The listing builds one solid part. Answer for the finished solid, in the listing's coordinates (mm). A direction names the side the tool comes from. Round coordinates to 2 decimals unless told otherwise and drop trailing zeros. Write each loop counter-clockwise with the first axis right and the second up, starting at its lowest first coordinate (ties: lowest second). Pieces come first, ordered by that corner, then holes. Notation, with made-up numbers: (34, 23) - (75, 23) arc R8 cw to (75, 38) - close; hole circle Ø2 at (18.25, 48). An arc over 180 degrees is marked (long way). Return JSON: item names as keys, results as strings. Group by question number.
(1) Each of these flat-tipped pins is pushed along its axis until it touches: pin 1 (2 mm diameter, centred on y = 131, z = 19, fed in from -X); pin 2 (5 mm diameter, centred on x = -15, z = 11.5, fed in from +Y); pin 3 (2 mm diameter, centred on x = -1.5, y = 134, fed in from -Z). Where does it stop, or does it pass through?
(2) Section A-A, the plane y = 120.5 is taken. Write down the section's boundary in (x, z).
(3) Which of the six approach directions +Z, -Z, +X, -X, +Y, -Y give full straight-line access (tool end or side, diameter ignored) to faces 4 (the flat face through (-16.028, 127.352, -1.676)), 5 (the cylindrical face through (-19.76, 136.28, -8.27)), 6 (the flat face through (-6.8, 127.5, 14.2))?
(4) Section B-B, the plane z = -0.5 is taken. Write down the section's boundary in (x, y).
(5) Determine the mould class of faces 1 (the cylindrical face through (-1, 120, 24)), 2 (the cylindrical face through (0.08, 119.36, 26.1)), 3 (the flat face through (-12, 136.799, 6)) for opening direction X: +X half, -X half, draft (parallel to the pull), parting line (faces both ways), or undercut.
(6) Section C-C, the plane y = 126.5 is taken. Write down the section's boundary in (x, z), then the cut area to 3 significant figures.
(7) Find the intervals of material crossed by line 1 along Y through (x, z) = (-17, -2); line 2 along X through (y, z) = (123.25, -8.5); line 3 along Y through (x, z) = (-19.25, -6), in increasing order. Write a range as [from, to].
(8) Section D-D, the plane x = -8.75 is taken. Write down the section's boundary in (y, z).
```python
from build123d import *

# Parameters (mm, degrees)
SKETCH1_R           = 2.15
BOSS_EXTRUDE1_DEPTH = 4.45
FILLET1_R           = 3


with BuildPart() as part:
    # Sketch1 → Boss-Extrude1 (new body)
    with BuildSketch(Plane(origin=(-13.195504222, 0, 7.618427915), x_dir=(0.5, 0, 0.866025404), z_dir=(-0.866025404, 0, 0.5))):
        Polygon((-25.134165871, 118.055853922), (-17.360832538, 136.798849573), (16.885834129, 136.798849573), (24.659167462, 118.055853922), align=None)
        with Locations((-13.360832538, 132.798849573)):
            Circle(SKETCH1_R, mode=Mode.SUBTRACT)
        with Locations((12.885834129, 132.798849573)):
            Circle(SKETCH1_R, mode=Mode.SUBTRACT)
        with Locations((19.659167462, 122.055853922)):
            Circle(SKETCH1_R, mode=Mode.SUBTRACT)
        with Locations((-20.134165871, 122.055853922)):
            Circle(SKETCH1_R, mode=Mode.SUBTRACT)
        Polygon((-12.804739093, 122.055853922), (-6.03140576, 132.798849573), (5.556407351, 132.798849573), (12.329740684, 122.055853922), align=None, mode=Mode.SUBTRACT)
    extrude(amount=-BOSS_EXTRUDE1_DEPTH)

    # Fillet1
    fillet1_edges = [part.edges().sort_by_distance(p)[0] for p in [
        (-23.835680634, 118.055853922, -15.260898232),
        (-19.949013967, 136.798849573, -8.528994094),
        (-2.825680634, 136.798849573, 21.129489235),
        (1.060986033, 118.055853922, 27.861393373),
    ]]
    fillet(fillet1_edges, radius=FILLET1_R)


solid = part.part
```
Working result:
{
 "1": {"pin 1": "stops at x = -7.19", "pin 2": "passes through", "pin 3": "stops at z = 17.58"},
 "2": {"outline": "(-24.99, -12.81) - (-21.14, -15.04) - (-20.15, -13.33) - (-24, -11.1) - close; (-22.52, -8.53) - (-18.67, -10.76) - (-0.25, 21.13) - (-4.11, 23.36) - close; (-2.62, 25.93) - (1.23, 23.7) - (2.22, 25.41) - (-1.64, 27.64) - close"},
 "3": {"face 4": "+Z, +X", "face 5": "-Z, -X, +Y", "face 6": "-Z, -X"},
 "4": {"outline": "(-17.88, 118.06) - (-12.74, 118.06) - (-12.74, 122.06) - (-17.88, 122.06) - close; (-17.88, 127.5) - (-12.74, 131.57) - (-12.74, 136.8) - (-17.88, 136.8) - close"},
 "5": {"face 1": "undercut", "face 2": "+X half", "face 3": "draft"},
 "6": {"outline": "(-24.01, -11.12) - (-20.16, -13.34) - (-14.34, -3.27) - (-18.2, -1.04) - close; (-8.43, 15.87) - (-4.58, 13.64) - (1.24, 23.72) - (-2.62, 25.94) - close", "area": "104 mm^2"},
 "7": {"line 1": "y = [118.06, 122.06], [126.14, 136.8]", "line 2": "x = [-21.97, -17.36]", "line 3": "y = [118.06, 131.22], [134.38, 136.8]"},
 "8": {"outline": "(118.06, 6.42) - (122.06, 6.42) - (122.06, 15.32) - (118.06, 15.32) - close; (127.51, 15.32) - (132.8, 11.47) - (132.8, 6.42) - (136.8, 6.42) - (136.8, 15.32) - close"}
}
